Geometry check sheet. Reference: the model listing, model coordinates, mm. Face numbers are marked on the shaded views. A direction names the side the tool comes from. Give positions to 0.01 mm unless a question says otherwise; leave off trailing zeros. Loops run counter-clockwise (first coordinate to the right, second up) from the corner with the lowest first, then second, coordinate; pieces in that order, holes last. Notation, with made-up numbers: (-7.5, 12.5) -> (-0.5, 12.5) arc R20 ccw to (-0.5, 31.5) -> close; hole circle Ø1 at (6, 81.25). An arc over 180 degrees is marked (long way). One line per question, with ' | ' between items.
from build123d import *

# Parameters (mm, degrees)
CROQUIS1_W              = 64
CROQUIS1_H              = 74
CROQUIS1_W_2            = 40
CROQUIS1_H_2            = 50
SALIENTE_EXTRUIR2_DEPTH = 25
SALIENTE_EXTRUIR3_DEPTH = 25
CORTAR_EXTRUIR1_REACH   = 143.863
CROQUIS3_R              = 6.5
REDONDEO1_R             = 12
REDONDEO2_R             = 12
CORTAR_EXTRUIR2_REACH   = 163.641


with BuildPart() as part:
    # Croquis1 → Saliente-Extruir2 (new body)
    with BuildSketch(Plane(origin=(0, 0, 0), x_dir=(1, 0, 0), z_dir=(0, 1, 0))):
        Rectangle(CROQUIS1_W, CROQUIS1_H)
        Rectangle(CROQUIS1_W_2, CROQUIS1_H_2, mode=Mode.SUBTRACT)
    extrude(amount=SALIENTE_EXTRUIR2_DEPTH)

    # Croquis2 → Saliente-Extruir3 (add, symmetric)
    with BuildSketch(Plane(origin=(0, 0, 0), x_dir=(0, 0, -1), z_dir=(1, 0, 0))):
        Polygon((37, 19), (53.784609691, 19), (115.951905284, 54.892304845), (121.951905284, 44.5), (57, 7), (37, 7), align=None)
        Polygon((-37, 19), (-57, 19), (-117.312425174, -15.821394909), (-111.312425174, -26.213699755), (-53.784609691, 7), (-37, 7), align=None)
    extrude(amount=SALIENTE_EXTRUIR3_DEPTH, both=True)

    # Croquis3 → Cortar-Extruir1 (cut, up to next)
    with BuildSketch(Plane(origin=(0, -9.039419162, -5.218911087), x_dir=(1, 0, 0), z_dir=(0, 0.8660254037844378, 0.5000000000000016)), mode=Mode.PRIVATE) as cortar_extruir1_sk1:
        with Locations(Location((-13, 115.863448016, 0), (0, 0, 270))):
            Circle(CROQUIS3_R)
    cortar_extruir1_tool1 = extrude(cortar_extruir1_sk1.sketch, amount=-CORTAR_EXTRUIR1_REACH, mode=Mode.PRIVATE) & part.part
    # Croquis3 → Cortar-Extruir1 (cut, up to next)
    with BuildSketch(Plane(origin=(0, -9.039419162, -5.218911087), x_dir=(1, 0, 0), z_dir=(0, 0.8660254037844378, 0.5000000000000016)), mode=Mode.PRIVATE) as cortar_extruir1_sk2:
        with Locations(Location((13, 115.863448016, 0), (0, 0, 270))):
            Circle(CROQUIS3_R)
    cortar_extruir1_tool2 = extrude(cortar_extruir1_sk2.sketch, amount=-CORTAR_EXTRUIR1_REACH, mode=Mode.PRIVATE) & part.part
    # Croquis3 → Cortar-Extruir1 (cut, up to next)
    with BuildSketch(Plane(origin=(0, -9.039419162, -5.218911087), x_dir=(1, 0, 0), z_dir=(0, 0.8660254037844378, 0.5000000000000016)), mode=Mode.PRIVATE) as cortar_extruir1_sk3:
        with Locations(Location((-13, 79.863448016, 0), (0, 0, 270))):
            Circle(CROQUIS3_R)
    cortar_extruir1_tool3 = extrude(cortar_extruir1_sk3.sketch, amount=-CORTAR_EXTRUIR1_REACH, mode=Mode.PRIVATE) & part.part
    # Croquis3 → Cortar-Extruir1 (cut, up to next)
    with BuildSketch(Plane(origin=(0, -9.039419162, -5.218911087), x_dir=(1, 0, 0), z_dir=(0, 0.8660254037844378, 0.5000000000000016)), mode=Mode.PRIVATE) as cortar_extruir1_sk4:
        with Locations(Location((13, 79.863448016, 0), (0, 0, 270))):
            Circle(CROQUIS3_R)
    cortar_extruir1_tool4 = extrude(cortar_extruir1_sk4.sketch, amount=-CORTAR_EXTRUIR1_REACH, mode=Mode.PRIVATE) & part.part
    add(cortar_extruir1_tool1.solids().sort_by_distance((-13, 48.892305, -105.5596))[0], mode=Mode.SUBTRACT)
    add(cortar_extruir1_tool2.solids().sort_by_distance((13, 48.892305, -105.5596))[0], mode=Mode.SUBTRACT)
    add(cortar_extruir1_tool3.solids().sort_by_distance((-13, 30.892305, -74.382686))[0], mode=Mode.SUBTRACT)
    add(cortar_extruir1_tool4.solids().sort_by_distance((13, 30.892305, -74.382686))[0], mode=Mode.SUBTRACT)

    # Redondeo1
    redondeo1_edges = [part.edges().sort_by_distance(p)[0] for p in [
        (25, -21.017547332, 114.312425174),
    ]]
    fillet(redondeo1_edges, radius=REDONDEO1_R)

    # Redondeo2
    redondeo2_edges = [part.edges().sort_by_distance(p)[0] for p in [
        (-25, -21.017547332, 114.312425174),
    ]]
    fillet(redondeo2_edges, radius=REDONDEO2_R)

    # Croquis5 → Cortar-Extruir2 (cut, up to next)
    with BuildSketch(Plane(origin=(0, 38.931724008, 22.477241336), x_dir=(1, 0, 0), z_dir=(0, 0.8660254037844378, 0.5000000000000016)), mode=Mode.PRIVATE) as cortar_extruir2_sk1:
        with BuildLine():
            Line((-10, -64.506237835), (-10, -109.506237835))
            Line((-10, -109.506237835), (10, -109.506237835))
            Line((10, -109.506237835), (10, -64.506237835))
            ThreePointArc((10, -64.506237835), (0, -54.506237835), (-10, -64.506237835))
        make_face()
    cortar_extruir2_tool1 = extrude(cortar_extruir2_sk1.sketch, amount=-CORTAR_EXTRUIR2_REACH, mode=Mode.PRIVATE) & part.part
    add(cortar_extruir2_tool1.solids().sort_by_distance((0, -2.584336, 94.385167))[0], mode=Mode.SUBTRACT)


solid = part.part
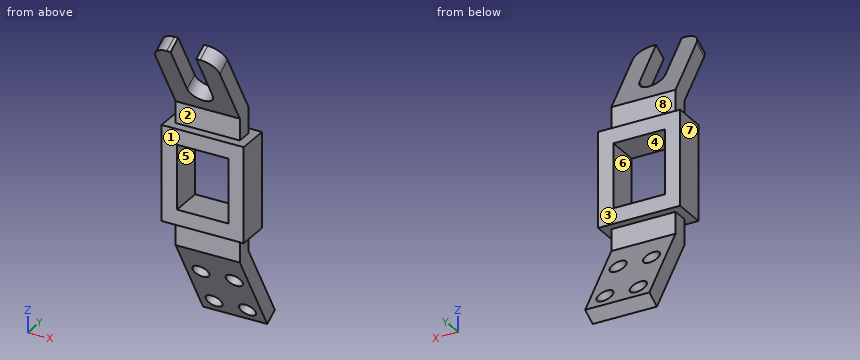
Item 1: Sectioned sample at C-C (z = 50). Record the cut outline in (x, y), plus the area to 3 significant figures.
Result:
outline: (-25, 7) -> (25, 7) -> (25, 19) -> (-25, 19) -> close | area: 600 mm2
Item 2: Release check for a two-part mould opening along X. For the marked faces 5, 6, 7 and 8 record: pulls with the +X half, pulls with the -X half, needs draft (parallel to the pull), parting line crosses it, or undercut.
Result:
face 5: undercut | face 6: undercut | face 7: pulls with the -X half | face 8: needs draft
Item 3: Scan lines: probe 1 along X at (y, z) = (0, 89); probe 2 along X at (y, z) = (21, -77); probe 3 along Z at (x, y) = (2.5, 23.5). Record each from-to range of solid material in increasing order.
Result:
probe 1: -25 to -10, 10 to 25 | probe 2: -25 to -18.92, -7.08 to 7.08, 18.92 to 25 | probe 3: -85.58 to -61.58, -37 to -25, 25 to 37
Item 4: Set-up check for the marked faces 1, 2, 3 and 4: record each of +Z, -Z, +X, -X, +Y, -Y from which the full face is reachable in a straight line by a thin tool's end or side.
Result:
face 1: -Z, +X, -X, -Y | face 2: +X, -X, -Y | face 3: +Z, +X, -X, +Y | face 4: +Y, -Y
Item 5: Sectioned sample at B-B (z = -78). Give the number of separate pieces and of enclosed holes in the cut face, plus the area to 3 significant figures.
Result:
separate pieces: 3 | enclosed holes: 0 | area: 353 mm2
Item 6: Sectioned sample at A-A (z = -11.5). Record the cut outline in (x, y), plus the area to 3 significant figures.
Result:
outline: (-32, 0) -> (-20, 0) -> (-20, 25) -> (-32, 25) -> close; (20, 0) -> (32, 0) -> (32, 25) -> (20, 25) -> close | area: 600 mm2
Item 7: Depth check by flat-ended pin: pin 1 Ø3 at (x, y) = (-11.5, 3) entering from -Z; pin 2 Ø7.5 at (x, y) = (10, 8) entering from +Z; pin 3 Ø10 at (y, z) = (-3, 104) entering from -X; pin 4 Ø2 at (y, z) = (27, 8) entering from +X. Enter the tip coordinate at first touch or a pass-through.
Result:
pin 1: z = -37 | pin 2: z = 82.55 | pin 3: x = -25 | pin 4: through
